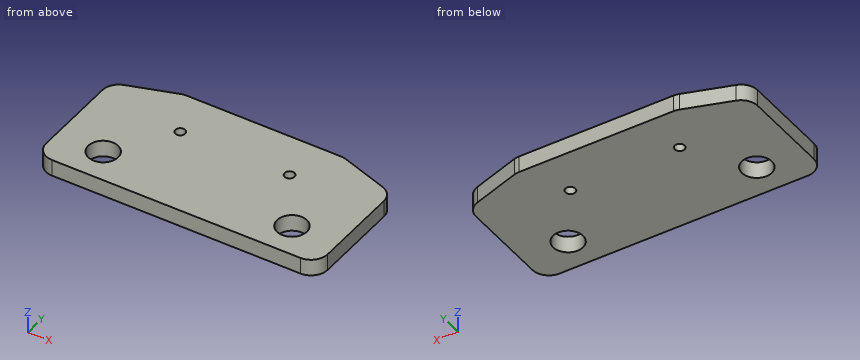
```python
from build123d import *

# Parameters (mm, degrees)
F0_R     = 4.5
F0_R_2   = 1.5
F1_DEPTH = 5


with BuildPart() as f1:
    # F0 (on Top) → F1 (new body)
    with BuildSketch(Plane.XY):
        with BuildLine():
            Line((-37.5, -27.5), (37.5, -27.5))
            ThreePointArc((37.5, -27.5), (41.035534, -26.035534), (42.5, -22.5))
            Line((42.5, -22.5), (42.5, 3.83017))
            ThreePointArc((42.5, 3.83017), (41.551788, 6.759848), (39.066796, 8.578344))
            Line((39.066796, 8.578344), (24.914882, 13.248173))
            ThreePointArc((24.914882, 13.248173), (24.141539, 13.436642), (23.348086, 13.5))
            Line((23.348086, 13.5), (0, 13.5))
            Line((0, 13.5), (-23.348086, 13.5))
            ThreePointArc((-23.348086, 13.5), (-24.141539, 13.436642), (-24.914882, 13.248173))
            Line((-24.914882, 13.248173), (-39.066796, 8.578344))
            ThreePointArc((-39.066796, 8.578344), (-41.551788, 6.759848), (-42.5, 3.83017))
            Line((-42.5, 3.83017), (-42.5, -22.5))
            ThreePointArc((-42.5, -22.5), (-41.035534, -26.035534), (-37.5, -27.5))
        make_face()
        with Locations((-28.5, -17.5)):
            Circle(F0_R, mode=Mode.SUBTRACT)
        with Locations((28.5, -17.5)):
            Circle(F0_R, mode=Mode.SUBTRACT)
        with Locations((-16.5, 0)):
            Circle(F0_R_2, mode=Mode.SUBTRACT)
        with Locations((16.5, 0)):
            Circle(F0_R_2, mode=Mode.SUBTRACT)
    extrude(amount=F1_DEPTH)


solid = f1.part
```
Input: part model. Units: mm. Frame: model coordinates. Round coordinates to 2 decimals unless told otherwise and drop trailing zeros. Loops run counter-clockwise (first coordinate to the right, second up) from the corner with the lowest first, then second, coordinate; pieces in that order, holes last. Notation, with made-up numbers: (-9, -15) - (13, -15) arc R22 ccw to (13, 3) - close; hole circle Ø6 at (89.25, -22.75). An arc over 180 degrees is marked (long way). One line per item, written item: value. Start each with the question number.
(1) Section C-C, the plane z = 3.1. Return loops of the section in (x, y), plus the area to 3 significant figures.
(2) Contact query for flat-ended pins moving along their axis: P1, Ø2, axis at x = -26, z = 1, coming from the +Y side; P2, Ø1.5, axis at x = 26.5, z = 4.5, coming from the +Y side; P3, Ø1, axis at y = 8, z = 3, coming from the +X side. Output: stop coordinate, or through.
(3) Section B-B, the plane y = -17.5. Return loops of the section in (x, z), plus the area to 3 significant figures.
(4) Section D-D, the plane y = 0. Return loops of the section in (x, z).
(5) Ray query, line 1 (X direction, y = -17, z = 2.2); line 2 (Y direction, x = -23.5, z = 1.6); line 3 (X direction, y = 0.5, z = 3.25). Return the intervals inside material, ascending. Write a range as [from, to].
(6) Section A-A, the plane x = -16.5. Return loops of the section in (y, z), plus the area to 3 significant figures.
Results below:
1. outline: (-42.5, -22.5) arc R5 ccw to (-37.5, -27.5) - (37.5, -27.5) arc R5 ccw to (42.5, -22.5) - (42.5, 3.83) arc R5 ccw to (39.07, 8.58) - (24.91, 13.25) arc R5 ccw to (23.35, 13.5) - (-23.35, 13.5) arc R5 ccw to (-24.91, 13.25) - (-39.07, 8.58) arc R5 ccw to (-42.5, 3.83) - close; hole circle Ø9 at (-28.5, -17.5); hole circle Ø3 at (-16.5, 0); hole circle Ø3 at (16.5, 0); hole circle Ø9 at (28.5, -17.5)
1. area: 3,220 mm^2
2. P1: y = 13.22
2. P2: y = 12.97
2. P3: x = 40.9
3. outline: (-42.5, 0) - (-33, 0) - (-33, 5) - (-42.5, 5) - close; (-24, 0) - (24, 0) - (24, 5) - (-24, 5) - close; (33, 0) - (42.5, 0) - (42.5, 5) - (33, 5) - close
3. area: 335 mm^2
4. outline: (-42.5, 0) - (-18, 0) - (-18, 5) - (-42.5, 5) - close; (-15, 0) - (15, 0) - (15, 5) - (-15, 5) - close; (18, 0) - (42.5, 0) - (42.5, 5) - (18, 5) - close
5. line 1: [-42.5, -32.97], [-24.03, 24.03], [32.97, 42.5]
5. line 2: [-27.5, 13.5]
5. line 3: [-42.5, -17.91], [-15.09, 15.09], [17.91, 42.5]
6. outline: (-27.5, 0) - (-1.5, 0) - (-1.5, 5) - (-27.5, 5) - close; (1.5, 0) - (13.5, 0) - (13.5, 5) - (1.5, 5) - close
6. area: 190 mm^2
